from build123d import *
from build123d.topology import SkipClean

# Parameters (mm, degrees)
SKETCH1_R           = 20
BOSS_EXTRUDE1_DEPTH = 40
SKETCH2_R           = 19
CUT_EXTRUDE1_DEPTH  = 39
BOSS_EXTRUDE2_START = -20
SKETCH5_R           = 2.5
SKETCH5_R_2         = 2.375
BOSS_EXTRUDE2_DEPTH = 40


with BuildPart() as part:
    # Sketch1 → Boss-Extrude1 (new body)
    with BuildSketch(Plane(origin=(0, 0, 0), x_dir=(1, 0, 0), z_dir=(0, 1, 0))):
        with Locations(Location((0, 0, 0), (0, 0, 270))):
            Circle(SKETCH1_R)
    extrude(amount=BOSS_EXTRUDE1_DEPTH)

    # Sketch2 → Cut-Extrude1 (cut)
    with BuildSketch(Plane(origin=(0, 40, 0), x_dir=(1, 0, 0), z_dir=(0, 1, 0))):
        with Locations(Location((0, 0, 0), (0, 0, 270))):
            Circle(SKETCH2_R)
    extrude(amount=-CUT_EXTRUDE1_DEPTH, mode=Mode.SUBTRACT)

    # Sketch5 → Boss-Extrude2 (add)
    with SkipClean():  # the faces are left unmerged after this step: merging them gives an invalid solid
        with BuildSketch(Plane(origin=(0, 0, 0), x_dir=(0, 0, -1), z_dir=(1, 0, 0)).offset(BOSS_EXTRUDE2_START)):
            with Locations(Location((0, 20, 0), (0, 0, 180))):
                Circle(SKETCH5_R)
            with Locations(Location((0, 20, 0), (0, 0, 180))):
                Circle(SKETCH5_R_2, mode=Mode.SUBTRACT)
        extrude(amount=BOSS_EXTRUDE2_DEPTH)


solid = part.part
CAD build for the part. Positions are in the model's coordinates, mm. A direction names the side the tool comes from. Round coordinates to 2 decimals unless told otherwise and drop trailing zeros. Order: outer loops, then holes, each group sorted by start corner. A loop starts at its lowest first (then second) coordinate and runs counter-clockwise, first axis right, second up. Notation, with made-up numbers: M 56.5,82.5 L 67.5,82.5 A24 ccw 67.5,99.5 Z; hole C 28.5,44.5 d9. An arc over 180 degrees is marked long. Use one line per item in the form item = value.
Q1. Probe L1, parallel to Y at x = 15, z = -6.5; L2, parallel to X at y = 17, z = 3.5; L3, parallel to X at y = 11, z = -3. List the from-to ranges inside material, lowest first.
Recorded:
L1 = 0 to 1
L2 = -19.69 to -18.67, 18.67 to 19.69
L3 = -19.77 to -18.76, 18.76 to 19.77
Q2. Saw through at D-D on y = 29. Give the cut face in (x, z).
Recorded:
outline = C 0,0 d40; hole C 0,0 d38
Q3. Which spindle directions (+Z, -Z, +X, -X, +Y, -Y) get a long thin tool onto all of the face, cutting with end or side? Do faces 5 (the flat face through (-7, 40, 18)), 6 (the cylindrical face through (-19, 20, 0)). Say none if no direction does.
Recorded:
face_5 = +Z, -Z, +X, -X, +Y
face_6 = none
Q4. Two-plate mould, pull along Z, no slides. Class faces 1 (the flat face through (0, 0, 0)), 2 (the cylindrical face through (19, 20, 0)), 3 (the cylindrical face through (-19.524, 19.72, -4.336)), 4 (the flat face through (0, 1, 0)): +Z half, -Z half, draft (parallel to the pull), parting line (faces both ways), or undercut.
Recorded:
face_1 = draft
face_2 = undercut
face_3 = parting line
face_4 = undercut
Q5. Saw through at B-B on x = -13.5. Give the cut face in (y, z) (3 decimals).
Recorded:
outline = M 0,-14.756 L 40,-14.756 L 40,-13.37 L 1,-13.37 L 1,13.37 L 40,13.37 L 40,14.756 L 0,14.756 Z; C 20,0 d5; hole C 20,0 d4.75
Q6. Saw through at C-C on z = -5. Give the cut face in (x, y).
Recorded:
outline = M -19.36,0 L 19.36,0 L 19.36,40 L 18.33,40 L 18.33,1 L -18.33,1 L -18.33,40 L -19.36,40 Z
Q7. Flat gauge pins, fed straight in: P1, Ø8, axis at y = 29.5, z = 3.5, coming from the +X side; P2, Ø1.5, axis at x = 14, z = 6, coming from the +Y side; P3, Ø2, axis at y = 18.5, z = 9, coming from the +X side; P4, Ø2, axis at x = 1.5, y = 20.5, coming from the +Z side. Where does each tip first touch, or does it go through?
Recorded:
P1 = 20
P2 = 1
P3 = 18.33
P4 = 19.99
Q8. Saw through at A-A on x = 11. Give the cut face in (y, z) (3 decimals), then the cut area to 3 significant figures.
Recorded:
outline = M 0,-16.703 L 40,-16.703 L 40,-15.492 L 1,-15.492 L 1,15.492 L 40,15.492 L 40,16.703 L 0,16.703 Z; C 20,0 d5; hole C 20,0 d4.75
area = 130 mm^2
